Answer from the drawing. Dimensions are ordinates in mm from the lowest x, y and z of the part. Coordinates: 2 decimals unless noted, no trailing zeros. Write each loop counter-clockwise with the first axis right and the second up, starting at its lowest first coordinate (ties: lowest second). Pieces come first, ordered by that corner, then holes.
(1) Section C-C on x = 49.5 is taken. Write down the section's boundary in (y, z), then the cut area to 3 significant figures.
(2) Find the intervals of material crossed by probe 1 along Z at (x, y) = (55.5, 1) (1 decimal); probe 2 along Z at (x, y) = (55, 3.8) (1 decimal); probe 3 along Z at (x, y) = (72, 3.5), in increasing order.
(3) Given pin 1 (2 mm diameter, centred on y = 2, z = 26, fed in from -X); pin 2 (3 mm diameter, centred on x = 78.38, z = 29.88, fed in from +Y); pin 3 (1 mm diameter, centred on y = 3.5, z = 55.5, fed in from +X) (1 decimal), each flat-ended and moving along its own axis, determine where each tip first touches the part or whether it passes through.
(4) Section A-A on z = 5 is taken. Write down the section's boundary in (x, y).
(5) Section B-B on y = 2.2 is taken. Write down the section's boundary in (x, z).
(6) Section D-D on z = 31 is taken. Write down the section's boundary in (x, y), then the cut area to 3 significant figures.
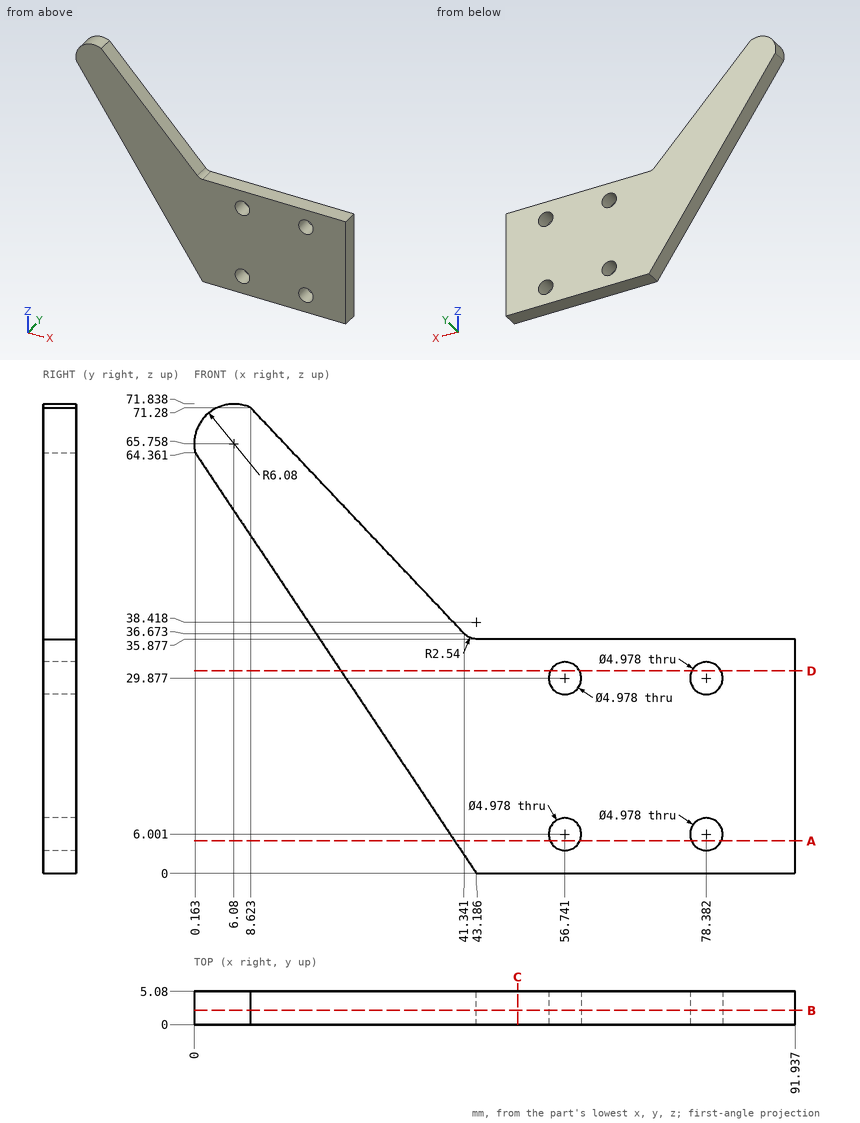
Response:
1. outline: (0, 0) - (5.08, 0) - (5.08, 35.88) - (0, 35.88) - close
1. area: 182 mm2
2. probe 1: z = 0 to 3.8, 8.2 to 27.7, 32 to 35.9
2. probe 2: z = 0 to 4.2, 7.8 to 28.1, 31.7 to 35.9
2. probe 3: z = 0 to 35.88
3. pin 1: stops at x = 25.14
3. pin 2: passes through
3. pin 3: stops at x = 24
4. outline: (39.84, 0) - (54.46, 0) - (54.46, 5.08) - (39.84, 5.08) - close; (59.02, 0) - (76.1, 0) - (76.1, 5.08) - (59.02, 5.08) - close; (80.66, 0) - (91.94, 0) - (91.94, 5.08) - (80.66, 5.08) - close
5. outline: (0.16, 64.36) - (43.19, 0) - (91.94, 0) - (91.94, 35.88) - (43.19, 35.88) arc R2.54 cw to (41.34, 36.67) - (8.62, 71.28) arc R6.08 ccw to start; hole circle Ø4.98 at (56.74, 6); hole circle Ø4.98 at (56.74, 29.88); hole circle Ø4.98 at (78.38, 6); hole circle Ø4.98 at (78.38, 29.88)
6. outline: (22.46, 0) - (54.52, 0) - (54.52, 5.08) - (22.46, 5.08) - close; (58.96, 0) - (76.16, 0) - (76.16, 5.08) - (58.96, 5.08) - close; (80.6, 0) - (91.94, 0) - (91.94, 5.08) - (80.6, 5.08) - close
6. area: 308 mm2
